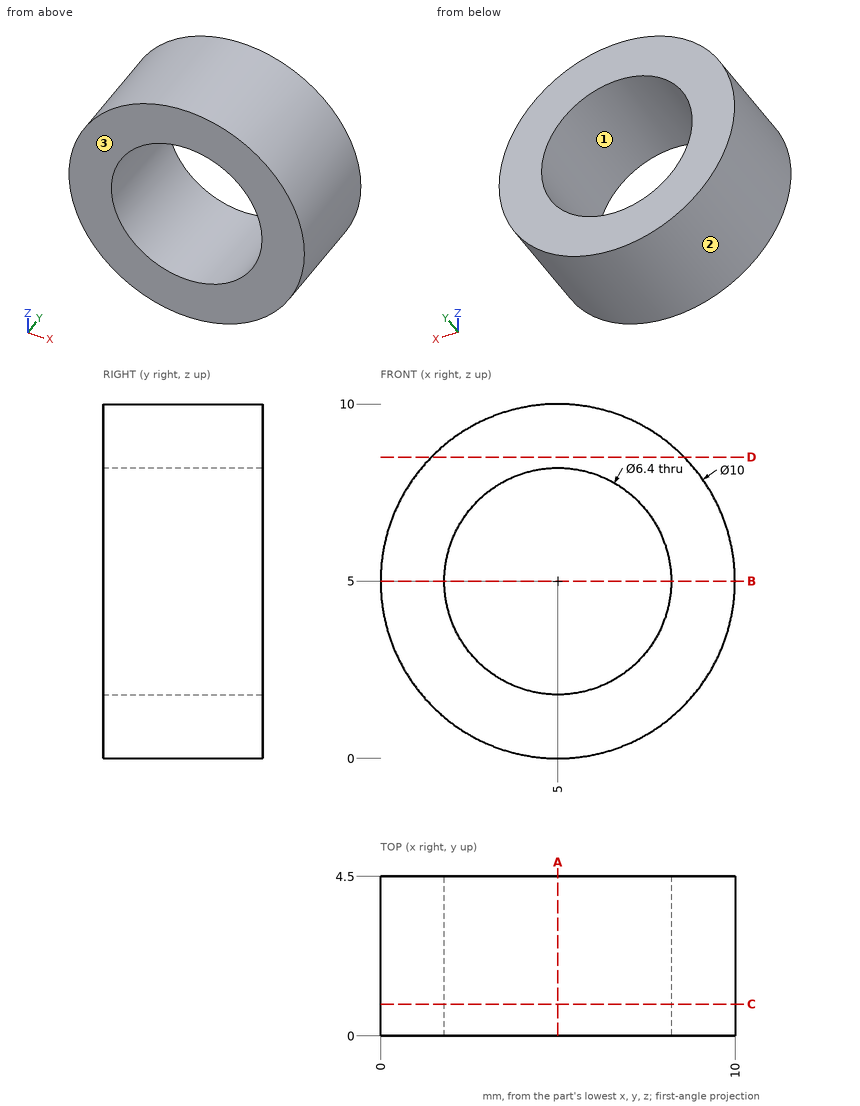
Source: three-view drawing plus pictorial views. Frame: mm from the lowest corner of the part. Give positions to 0.01 mm unless a question says otherwise; leave off trailing zeros. Loops run counter-clockwise (first coordinate to the right, second up) from the corner with the lowest first, then second, coordinate; pieces in that order, holes last. Notation, with made-up numbers: M -15.75,79.5 L -6.75,79.5 A25 cw -6.75,113.5 Z; hole C 28.5,57.5 d11. An arc over 180 degrees is marked long. Put each result on its own line as item: value.
Q1. Mould query, pull axis X, two halves, no side actions, for the marked faces 1, 2 and 3. Classes: released by +X, released by -X, zero draft, split by the parting line, or undercut.
Response values:
face 1: undercut
face 2: split by the parting line
face 3: zero draft
Q2. Line query: probe 1 along Z at (x, y) = (5, 0.95); probe 2 along X at (y, z) = (4, 2.25); probe 3 along Z at (x, y) = (7.25, 3.15). Output: solid intervals per line, ascending. Write a range as [from, to].
Response values:
probe 1: z = [0, 1.8], [8.2, 10]
probe 2: x = [0.82, 3.36], [6.64, 9.18]
probe 3: z = [0.53, 2.72], [7.28, 9.47]
Q3. Section D-D (z = 8.5). Return the cut outline in (x, y).
Response values:
outline: M 1.43,0 L 8.57,0 L 8.57,4.5 L 1.43,4.5 Z
Q4. Section C-C (y = 0.9). Return the cut outline in (x, z), and give its area (3 significant figures).
Response values:
outline: C 5,5 d10; hole C 5,5 d6.4
area: 46.4 mm²
Q5. Section B-B (z = 5). Return the cut outline in (x, y).
Response values:
outline: M 0,0 L 1.8,0 L 1.8,4.5 L 0,4.5 Z; M 8.2,0 L 10,0 L 10,4.5 L 8.2,4.5 Z
Q6. Section A-A (x = 5). Return the cut outline in (y, z), and give its area (3 significant figures).
Response values:
outline: M 0,0 L 4.5,0 L 4.5,1.8 L 0,1.8 Z; M 0,8.2 L 4.5,8.2 L 4.5,10 L 0,10 Z
area: 16.2 mm²
